Verification items for the finished model (mm, model axes). A direction names the side the tool comes from. Give positions to 0.01 mm unless a question says otherwise; leave off trailing zeros. Loops run counter-clockwise (first coordinate to the right, second up) from the corner with the lowest first, then second, coordinate; pieces in that order, holes last. Notation, with made-up numbers: (77, 34) -> (117, 34) arc R31 ccw to (117, 67) -> close; hole circle Ø8 at (-38, 80.5). An arc over 180 degrees is marked (long way). Answer in a Markdown table with one row per item. Add a question column.
Q1. Material ranges on probe 1 along Y at (x, z) = (5, -0.75); probe 2 along Y at (x, z) = (5.5, -1); probe 3 along Z at (x, y) = (8.75, -7.75), recorded low to high.
Q2. Release check for a two-part mould opening along X. For faces 4 (the face through (12.932, 5.362, -6.386)), 5 (the face through (3.581, -3.547, -1.914)), 6 (the face through (-7, 0, 0)), 7 (the face through (-3, 9, -7.4)) record: pulls with the +X half, pulls with the -X half, needs draft (parallel to the pull), parting line crosses it, or undercut.
Q3. Section check B-B on z = 0.75. Enter the section's corners in (x, y).
Q4. Section check D-D on y = 8.25. Enter the section's corners in (x, z).
Q5. Set-up check for faces 1 (the face through (-0.041, -3.732, 0.913)), 2 (the face through (-6.567, 2.494, 0.913)), 3 (the face through (0, 4, -2.9)): record each of +Z, -Z, +X, -X, +Y, -Y from which the full face is reachable in a straight line by a thin tool's end or side.
Q6. Gauge pin test, flat ends, axial feed: P1, Ø4.5, axis at x = 0, y = 0, coming from the +Z side; P2, Ø3.5, axis at x = 4.31, y = -5.52, coming from the +Z side; P3, Ø2.5, axis at x = -4.31, y = 5.52, coming from the -Z side; P4, Ø4, axis at y = 7.5, z = -5.5, coming from the -X side. Record the tip position at first contact, or that the pin passes through.
Q7. Section check C-C on y = 0. Enter the section's corners in (x, z), and give its area (4 significant figures).
```python
from build123d import *

# Parameters (mm, degrees)
BOSS_EXTRU_1_START      = 1.8
ESQUISSE2_R             = 0.5
BOSS_EXTRU_1_DEPTH      = 1.8
ESQUISSE4_R             = 0.5
ENL_V_MAT_EXTRU_3_DEPTH = 22.832086478
ESQUISSE6_R             = 2.1
ENL_V_MAT_EXTRU_4_DEPTH = 2
ESQUISSE7_R             = 1.05
ENL_V_MAT_EXTRU_5_DEPTH = 21.349201459


with BuildPart() as part:
    # Esquisse1 → R_volution1 (revolve)
    with BuildSketch(Plane(origin=(0, 0, 0), x_dir=(1, 0, 0), z_dir=(0, 1, 0)), mode=Mode.PRIVATE) as r_volution1_sk:
        Polygon((-11, 0), (-3.75, 0), (-3.75, 2.9), (-9, 2.9), (-9, 7.4), (-14, 7.4), (-14, 5.4), (-11, 5.4), align=None)
    revolve(r_volution1_sk.sketch.rotate(Axis((0, 0, 0), (0, 0, -1)), 180), axis=Axis((0, 0, 0), (0, 0, -1)))

    # Esquisse2 → Boss.-Extru.1 (add)
    with BuildSketch(Plane.XY.offset(BOSS_EXTRU_1_START)):
        with Locations(Location((-8.872610569, 0, 0), (0, 0, 180))):
            Circle(ESQUISSE2_R)
        with Locations(Location((8.927389431, 0, 0), (0, 0, 180))):
            Circle(ESQUISSE2_R)
        with BuildLine():
            Line((-2.468322158, 2.8), (-10.781965021, 2.179272878))
            ThreePointArc((-10.781965021, 2.179272878), (-0.002117582, 10.999999796), (10.78112517, 2.183423933))
            Line((10.78112517, 2.183423933), (2.463250179, 2.804463021))
            ThreePointArc((2.463250179, 2.804463021), (-0.003378, 3.732640201), (-2.468322158, 2.8))
        make_face()
        with BuildLine():
            Line((-10.781965021, -2.179272878), (-2.468322158, -2.8))
            ThreePointArc((-2.468322158, -2.8), (-0.003378, -3.732640201), (2.463250179, -2.804463021))
            Line((2.463250179, -2.804463021), (10.78112517, -2.183423933))
            ThreePointArc((10.78112517, -2.183423933), (-0.002117582, -10.999999796), (-10.781965021, -2.179272878))
        make_face()
    extrude(amount=-BOSS_EXTRU_1_DEPTH)

    # Esquisse4 → Enl_v. mat.-Extru.3 (cut, through all)
    with BuildSketch(Plane.XY.offset(1.8)):
        with Locations(Location((-8.872610569, 0, 0), (0, 0, 103.20473155))):
            Circle(ESQUISSE4_R)
        with Locations(Location((8.927389431, 0, 0), (0, 0, 83.234386781))):
            Circle(ESQUISSE4_R)
    extrude(amount=-ENL_V_MAT_EXTRU_3_DEPTH, mode=Mode.SUBTRACT)

    # Esquisse6 → Enl_v. mat.-Extru.4 (cut)
    with BuildSketch(Plane(origin=(0, 0, -2.9), x_dir=(-1, 0, 0), z_dir=(0, 0, -1))):
        with Locations((-4.309630327, 5.516075275)):
            Circle(ESQUISSE6_R)
        with Locations(Location((4.309630327, 5.516075275, 0), (0, 0, 31.79043646))):
            Circle(ESQUISSE6_R)
        with Locations(Location((-4.309630327, -5.516075275, 0), (0, 0, 252.20956354))):
            Circle(ESQUISSE6_R)
        with Locations((4.309630327, -5.516075275)):
            Circle(ESQUISSE6_R)
    extrude(amount=-ENL_V_MAT_EXTRU_4_DEPTH, mode=Mode.SUBTRACT)

    # Esquisse7 → Enl_v. mat.-Extru.5 (cut, through all)
    with BuildSketch(Plane(origin=(0, 0, -2.9), x_dir=(-1, 0, 0), z_dir=(0, 0, -1))):
        with Locations((4.309630327, -5.516075275)):
            Circle(ESQUISSE7_R)
        with Locations(Location((-4.309630327, -5.516075275, 0), (0, 0, 180))):
            Circle(ESQUISSE7_R)
        with Locations(Location((4.309630327, 5.516075275, 0), (0, 0, 180))):
            Circle(ESQUISSE7_R)
        with Locations((-4.309630327, 5.516075275)):
            Circle(ESQUISSE7_R)
    extrude(amount=-ENL_V_MAT_EXTRU_5_DEPTH, mode=Mode.SUBTRACT)


solid = part.part
```
Taken from the geometry:
| question | item | result |
|---|---|---|
| 1 | probe 1 | y = -9.8 to -6.31, -4.72 to 4.72, 6.31 to 9.8 |
| 1 | probe 2 | y = -9.53 to -7.25, -3.79 to 3.79, 7.25 to 9.53 |
| 1 | probe 3 | z = -7.4 to -5.4 |
| 2 | face 4 | parting line crosses it |
| 2 | face 5 | undercut |
| 2 | face 6 | undercut |
| 2 | face 7 | needs draft |
| 3 | outline | (-10.78, -2.18) arc R11 ccw to (10.78, -2.18) -> (2.46, -2.8) arc R3.73 cw to (-2.47, -2.8) -> close; (-10.78, 2.18) -> (-2.47, 2.8) arc R3.73 cw to (2.46, 2.8) -> (10.78, 2.18) arc R11 ccw to start; hole circle Ø2.1 at (-4.31, -5.52); hole circle Ø2.1 at (-4.31, 5.52); hole circle Ø2.1 at (4.31, -5.52); hole circle Ø2.1 at (4.31, 5.52) |
| 4 | outline | (-11.31, -7.4) -> (-3.6, -7.4) -> (-3.6, -2.9) -> (3.6, -2.9) -> (3.6, -7.4) -> (11.31, -7.4) -> (11.31, -5.4) -> (7.28, -5.4) -> (7.28, 1.8) -> (-7.28, 1.8) -> (-7.28, -5.4) -> (-11.31, -5.4) -> close |
| 5 | face 1 | +Z, -Z |
| 5 | face 2 | +Z |
| 5 | face 3 | -Z |
| 6 | P1 | passes through |
| 6 | P2 | stops at z = 1.8 |
| 6 | P3 | stops at z = -0.9 |
| 6 | P4 | stops at x = -12.87 |
| 7 | outline | (-14, -7.4) -> (-9.37, -7.4) -> (-9.37, 0) -> (-11, 0) -> (-11, -5.4) -> (-14, -5.4) -> close; (-8.37, -2.9) -> (-3.75, -2.9) -> (-3.75, 0) -> (-8.37, 0) -> close; (3.75, -2.9) -> (8.43, -2.9) -> (8.43, 0) -> (3.75, 0) -> close; (9.43, -7.4) -> (14, -7.4) -> (14, -5.4) -> (11, -5.4) -> (11, 0) -> (9.43, 0) -> close |
| 7 | area | 62.65 mm² |
